Drawing for the job (mm, zero at the part's lowest x, y, z). A direction names the side the tool comes from. Round coordinates to 2 decimals unless told otherwise and drop trailing zeros. Loops run counter-clockwise (first coordinate to the right, second up) from the corner with the lowest first, then second, coordinate; pieces in that order, holes last. Notation, with made-up numbers: M -7.5,-22.5 L 9.5,-22.5 A11 ccw 9.5,-5.5 Z; hole C 52,62.25 d10. An arc over 180 degrees is marked long. Answer in a Markdown table with one row per item.
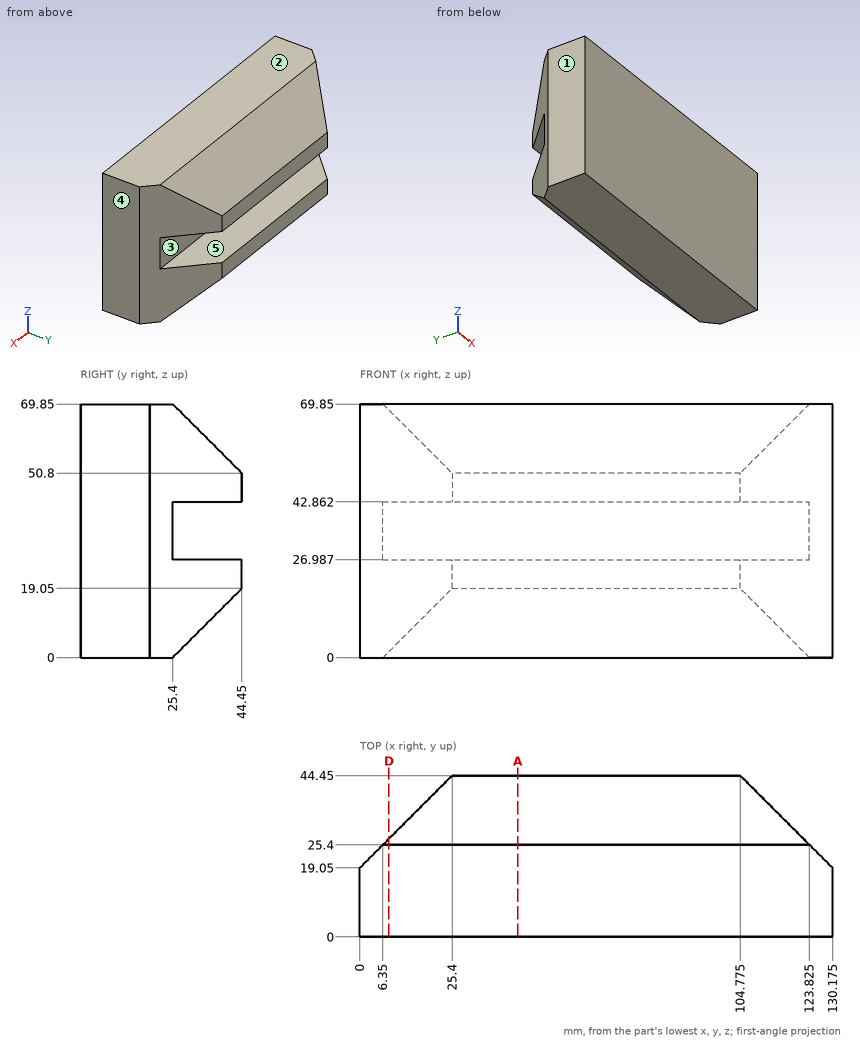
1. Wall check: probe 1 along Y at (x, z) = (104.5, 36.5); probe 2 along Y at (x, z) = (107.5, 56.5). Give the ranges that are in metal, low to high.
Verdict:
| item | result |
|---|---|
| probe 1 | y = 0 to 25.4 |
| probe 2 | y = 0 to 38.75 |
2. Saw through at A-A (x = 43.5). Write the cut outline in (y, z).
Verdict:
| item | result |
|---|---|
| outline | M 0,0 L 25.4,0 L 44.45,19.05 L 44.45,26.99 L 25.4,26.99 L 25.4,42.86 L 44.45,42.86 L 44.45,50.8 L 25.4,69.85 L 0,69.85 Z |
3. Tool access for the marked faces 4 and 5: list every direction of +Z, -Z, +X, -X, +Y, -Y with a clear straight run to the whole face (end or side of a thin tool).
Verdict:
| item | result |
|---|---|
| face 4 | +Z, -Z, +X, +Y, -Y |
| face 5 | +X, -X, +Y |
4. Mould opens along Z. For the marked faces 1, 2 and 3 say: +Z half, -Z half, draft (parallel to the pull), parting line (faces both ways), or undercut.
Verdict:
| item | result |
|---|---|
| face 1 | draft |
| face 2 | +Z half |
| face 3 | undercut |
5. Pin check, flat tips, straight feed: pin 1 (8 mm diameter, centred on x = 43.5, z = 14, fed in from +Y); pin 2 (5.5 mm diameter, centred on x = 50, y = 38, fed in from -Z); pin 3 (4 mm diameter, centred on y = 39, z = 44.5, fed in from +X) (1 decimal). Stop position of each tip, or through.
Verdict:
| item | result |
|---|---|
| pin 1 | stops at y = 43.4 |
| pin 2 | stops at z = 9.85 |
| pin 3 | stops at x = 112.2 |
6. Saw through at D-D (x = 8). Write the cut outline in (y, z).
Verdict:
| item | result |
|---|---|
| outline | M 0,0 L 25.4,0 L 27.05,1.65 L 27.05,26.99 L 25.4,26.99 L 25.4,42.86 L 27.05,42.86 L 27.05,68.2 L 25.4,69.85 L 0,69.85 Z |
